```python
from build123d import *

# Parameters (mm, degrees)
SKETCH1_R           = 18.5
SKETCH1_R_2         = 15
BOSS_EXTRUDE1_DEPTH = 4
SKETCH2_R           = 17.5
SKETCH2_R_2         = 16
CUT_EXTRUDE1_DEPTH  = 1
CUT_EXTRUDE2_START  = -1
SKETCH3_R           = 17.5
SKETCH3_R_2         = 16
CUT_EXTRUDE2_DEPTH  = 1
CHAMFER1_SIZE       = 0.2


with BuildPart() as part:
    # Sketch1 → Boss-Extrude1 (new body)
    with BuildSketch(Plane(origin=(0, 0, 0), x_dir=(1, 0, 0), z_dir=(0, 1, 0))):
        with Locations(Location((0, 0, 0), (0, 0, 270))):
            Circle(SKETCH1_R)
        with Locations(Location((0, 0, 0), (0, 0, 270))):
            Circle(SKETCH1_R_2, mode=Mode.SUBTRACT)
    extrude(amount=BOSS_EXTRUDE1_DEPTH)

    # Sketch2 → Cut-Extrude1 (cut)
    with BuildSketch(Plane(origin=(0, 4, 0), x_dir=(1, 0, 0), z_dir=(0, 1, 0))):
        with Locations(Location((0, 0, 0), (0, 0, 270))):
            Circle(SKETCH2_R)
        with Locations(Location((0, 0, 0), (0, 0, 270))):
            Circle(SKETCH2_R_2, mode=Mode.SUBTRACT)
    extrude(amount=-CUT_EXTRUDE1_DEPTH, mode=Mode.SUBTRACT)

    # Sketch3 → Cut-Extrude2 (cut)
    with BuildSketch(Plane.XZ.offset(CUT_EXTRUDE2_START)):
        with Locations(Location((0, 0, 0), (0, 0, 90))):
            Circle(SKETCH3_R)
        with Locations(Location((0, 0, 0), (0, 0, 90))):
            Circle(SKETCH3_R_2, mode=Mode.SUBTRACT)
    extrude(amount=CUT_EXTRUDE2_DEPTH, mode=Mode.SUBTRACT)

    # Chamfer1
    chamfer1_edges = [part.edges().sort_by_distance(p)[0] for p in [
        (0, 4, -17.5),
        (0, 4, -16),
        (0, 0, -18.5),
        (0, 0, -17.5),
        (0, 0, -16),
        (0, 4, -18.5),
        (0, 0, -15),
        (0, 4, -15),
    ]]
    chamfer(chamfer1_edges, length=CHAMFER1_SIZE)


solid = part.part
```
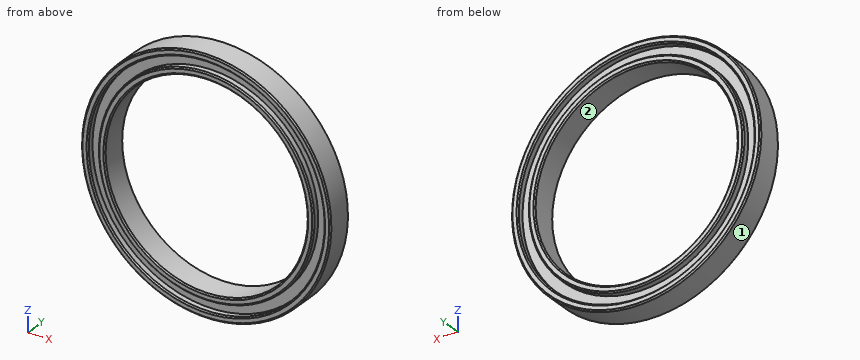
Build history of the part. All positions in model axes, mm. Face numbers are marked on the shaded views. Coordinates: 2 decimals unless noted, no trailing zeros. Order: outer loops, then holes, each group sorted by start corner. A loop starts at its lowest first (then second) coordinate and runs counter-clockwise, first axis right, second up.
Item 1: Saw through at A-A on y = 1.6. List the corners of the cut face in (x, z).
Filled in:
outline: circle Ø37 at (0, 0); hole circle Ø30 at (0, 0)
Item 2: Drop flat-ended pins along their axis: pin 1 Ø1 at (y, z) = (3, -7) entering from -X; pin 2 Ø2 at (y, z) = (0.5, 2.5) entering from +X. Give the stop position or say it passes through.
Filled in:
pin 1: stops at x = -17.32
pin 2: stops at x = 18.44
Item 3: Mould opens along X. For the marked faces 1 and 2 say: released by +X, released by -X, zero draft, split by the parting line, or undercut.
Filled in:
face 1: split by the parting line
face 2: undercut
Item 4: Drill centre lines: L1, parallel to X at y = 0.75, z = 0; L2, parallel to X at y = 2.3, z = 0; L3, parallel to Z at x = 0.5, y = 0.3. Where is each one in solid material? Low to high.
Filled in:
L1: x = -18.5 to -17.5, -16 to -15, 15 to 16, 17.5 to 18.5
L2: x = -18.5 to -15, 15 to 18.5
L3: z = -18.49 to -17.49, -15.99 to -14.99, 14.99 to 15.99, 17.49 to 18.49
